from build123d import *

# Parameters (mm, degrees)
SKETCH1_R                = 200
BOSS_EXTRUDE1_DEPTH      = 15
BOSS_EXTRUDE2_DEPTH      = 200
CUT_EXTRUDE1_DEPTH       = 286.087705803
CUT_EXTRUDE1_DEPTH_BACK  = 286.087705803
SKETCH3_R                = 85
CUT_EXTRUDE2_DEPTH       = 451.079120005
CUT_EXTRUDE2_DEPTH_BACK  = 451.079120005
SKETCH4_R                = 11
CUT_EXTRUDE3_DEPTH       = 451.079120105
CUT_EXTRUDE3_DEPTH_BACK  = 110
CUT_EXTRUDE4_DEPTH       = 110
BOSS_EXTRUDE3_DEPTH      = 200
CUT_EXTRUDE5_DEPTH       = 286.087705815
CUT_EXTRUDE5_DEPTH_BACK  = 286.087705815
SKETCH7_OUTSIDE_W        = 515.59
SKETCH7_OUTSIDE_H        = 515.59
SKETCH7_OUTSIDE_R        = 200
SKETCH9_R                = 5.9
BOSS_EXTRUDE4_DEPTH      = 230
CUT_EXTRUDE6_DEPTH       = 190
CUT_EXTRUDE8_DEPTH       = 307.879455313
CUT_EXTRUDE8_DEPTH_BACK  = 307.879455313
SKETCH12_OUTSIDE_W       = 584.34
SKETCH12_OUTSIDE_H       = 524.34
SKETCH12_OUTSIDE_W_2     = 160.728506479
SKETCH12_OUTSIDE_H_2     = 57.445626466
BOSS_EXTRUDE5_DEPTH      = 190
CUT_EXTRUDE10_DEPTH      = 198.357534097
CUT_EXTRUDE10_DEPTH_BACK = 198.357534097
SKETCH20_W               = 10
SKETCH20_H               = 6
BOSS_EXTRUDE6_DEPTH      = 200
CUT_EXTRUDE9_DEPTH       = 237.718926518
CUT_EXTRUDE9_DEPTH_BACK  = 237.718926518
SKETCH15_R               = 85
CUT_EXTRUDE11_START      = 4.5
CUT_EXTRUDE11_DEPTH      = 6
CUT_EXTRUDE12_DEPTH      = 10
CUT_EXTRUDE13_DEPTH      = 10
SKETCH25_R               = 2.75
CUT_EXTRUDE14_DEPTH      = 100
SKETCH26_R               = 3.05
CUT_EXTRUDE15_DEPTH      = 12.1
FILLET1_R                = 5
CUT_EXTRUDE16_DEPTH      = 3
LPATTERN1_COUNT          = 3
LPATTERN1_PITCH          = 30
CUT_EXTRUDE17_DEPTH      = 3
LPATTERN2_COUNT          = 3
LPATTERN2_PITCH          = 30
BOSS_EXTRUDE7_START      = 12.1
BOSS_EXTRUDE7_DEPTH      = 12.1


# Read off the part's stored shape, not the designer's step: Cut-Extrude11
with BuildPart() as part:
    # Sketch1 → Boss-Extrude1 (new body)
    with BuildSketch(Plane(origin=(0, 0, 0), x_dir=(1, 0, 0), z_dir=(0, 1, 0))):
        with Locations(Location((0, 0, 0), (0, 0, 270))):
            Circle(SKETCH1_R)
    extrude(amount=BOSS_EXTRUDE1_DEPTH)

    # Sketch2 → Boss-Extrude2 (add, symmetric)
    with BuildSketch(Plane.XY):
        Polygon((-25, 50.707142143), (25, 50.707142143), (60, 15), (-60, 15), align=None)
    extrude(amount=BOSS_EXTRUDE2_DEPTH, both=True)

    # Sketch3 → Cut-Extrude1 (cut, two sides: drawn at the far end of the back side and taken through both)
    with BuildSketch(Plane(origin=(0, 15, 0), x_dir=(1, 0, 0), z_dir=(0, 1, 0)).offset(-CUT_EXTRUDE1_DEPTH_BACK)):
        with Locations(Location((0, 0, 0), (0, 0, 270))):
            Circle(SKETCH3_R)
    extrude(amount=CUT_EXTRUDE1_DEPTH + CUT_EXTRUDE1_DEPTH_BACK, mode=Mode.SUBTRACT)

    # Sketch4 → Cut-Extrude2 (cut, two sides: drawn at the far end of the back side and taken through both)
    with BuildSketch(Plane(origin=(0, 0, -200), x_dir=(-1, 0, 0), z_dir=(0, 0, -1)).offset(-CUT_EXTRUDE2_DEPTH_BACK)):
        with Locations((0, 29)):
            Circle(SKETCH4_R)
    extrude(amount=CUT_EXTRUDE2_DEPTH + CUT_EXTRUDE2_DEPTH_BACK, mode=Mode.SUBTRACT)

    # Sketch5 → Cut-Extrude3 (cut, two sides: drawn at the far end of the back side and taken through both)
    with BuildSketch(Plane.XY.offset(200).offset(-CUT_EXTRUDE3_DEPTH_BACK)):
        Polygon((-25, 50.707142143), (25, 50.707142143), (50.198039412, 25), (25, 25), (25, 15), (-25, 15), (-25, 25), (-50.198039412, 25), align=None)
    extrude(amount=CUT_EXTRUDE3_DEPTH + CUT_EXTRUDE3_DEPTH_BACK, mode=Mode.SUBTRACT)

    # Sketch6 → Cut-Extrude4 (cut)
    with BuildSketch(Plane(origin=(0, 0, -200), x_dir=(-1, 0, 0), z_dir=(0, 0, -1))):
        Polygon((-25, 50.707142143), (25, 50.707142143), (50.198039412, 25), (25, 25), (25, 15), (-25, 15), (-25, 25), (-50.198039412, 25), align=None)
    extrude(amount=-CUT_EXTRUDE4_DEPTH, mode=Mode.SUBTRACT)

    # Sketch8 → Boss-Extrude3 (add, symmetric)
    with BuildSketch(Plane(origin=(0, 0, 0), x_dir=(0, 0, -1), z_dir=(1, 0, 0))):
        Polygon((0, 15), (-30, 15), (-29.95, 44.999958333), (29.95, 44.999958333), (30, 15), align=None)
    extrude(amount=BOSS_EXTRUDE3_DEPTH, both=True)

    # Sketch7 outside → Cut-Extrude5 (cut, two sides: drawn at the far end of the back side and taken through both)
    with BuildSketch(Plane(origin=(0, 15, 0), x_dir=(1, 0, 0), z_dir=(0, 1, 0)).offset(-CUT_EXTRUDE5_DEPTH_BACK)):
        Rectangle(SKETCH7_OUTSIDE_W, SKETCH7_OUTSIDE_H)
        with Locations(Location((0, 0, 0), (0, 0, 97.180755781))):
            Circle(SKETCH7_OUTSIDE_R, mode=Mode.SUBTRACT)
    extrude(amount=CUT_EXTRUDE5_DEPTH + CUT_EXTRUDE5_DEPTH_BACK, mode=Mode.SUBTRACT)

    # Sketch9 → Boss-Extrude4 (add, symmetric)
    with BuildSketch(Plane(origin=(0, 0, 0), x_dir=(0, 0, -1), z_dir=(1, 0, 0))):
        with Locations(Location((0, 29, 0), (0, 0, 180))):
            Circle(SKETCH9_R)
    extrude(amount=BOSS_EXTRUDE4_DEPTH, both=True)

    # Sketch10 → Cut-Extrude6 (cut, symmetric)
    with BuildSketch(Plane(origin=(0, 0, 0), x_dir=(0, 0, -1), z_dir=(1, 0, 0))):
        Polygon((-30, 15), (30, 15), (29.95, 44.999958333), (-29.95, 44.999958333), align=None)
    extrude(amount=CUT_EXTRUDE6_DEPTH, both=True, mode=Mode.SUBTRACT)

    # Sketch12 outside → Cut-Extrude8 (cut, two sides: drawn at the far end of the back side and taken through both)
    with BuildSketch(Plane(origin=(0, 15, 0), x_dir=(1, 0, 0), z_dir=(0, 1, 0)).offset(-CUT_EXTRUDE8_DEPTH_BACK)):
        Rectangle(SKETCH12_OUTSIDE_W, SKETCH12_OUTSIDE_H)
        with Locations((-160.364253239, 0)):
            Rectangle(SKETCH12_OUTSIDE_W_2, SKETCH12_OUTSIDE_H_2, mode=Mode.SUBTRACT)
    extrude(amount=CUT_EXTRUDE8_DEPTH + CUT_EXTRUDE8_DEPTH_BACK, mode=Mode.SUBTRACT)

    # Sketch14 → Boss-Extrude5 (add)
    with BuildSketch(Plane(origin=(0, 0, 0), x_dir=(0, 0, -1), z_dir=(1, 0, 0))):
        Polygon((-28.722813233, 15), (-28.722813233, 35), (-18.722813233, 35), (-18.722813233, 25), (-10.722813233, 15), align=None)
        Polygon((28.722813233, 15), (28.722813233, 35), (18.722813233, 35), (18.722813233, 25), (10.722813233, 15), align=None)
    extrude(amount=-BOSS_EXTRUDE5_DEPTH)

    # Sketch16 → Cut-Extrude10 (cut, two sides: drawn at the far end of the back side and taken through both)
    with BuildSketch(Plane(origin=(-190, 0, 0), x_dir=(0, 0, -1), z_dir=(1, 0, 0)).offset(-CUT_EXTRUDE10_DEPTH_BACK)):
        Polygon((-28.722813233, 35), (-10.596657492, 40.452365235), (10.596657492, 40.452365235), (28.722813233, 35), (31.38249, 46.365203084), (-30.991256821, 46.365203084), align=None)
    extrude(amount=CUT_EXTRUDE10_DEPTH + CUT_EXTRUDE10_DEPTH_BACK, mode=Mode.SUBTRACT)

    # Sketch20 → Boss-Extrude6 (add)
    with BuildSketch(Plane(origin=(0, 0, 0), x_dir=(0, 0, -1), z_dir=(1, 0, 0))):
        with Locations((-33.722813233, 7.5)):
            Rectangle(SKETCH20_W, SKETCH20_H)
        with Locations((33.722813233, 7.5)):
            Rectangle(SKETCH20_W, SKETCH20_H)
    extrude(amount=-BOSS_EXTRUDE6_DEPTH)

    # Sketch15 → Cut-Extrude9 (cut, two sides: drawn at the far end of the back side and taken through both)
    with BuildSketch(Plane(origin=(0, 0, 0), x_dir=(1, 0, 0), z_dir=(0, 1, 0)).offset(-CUT_EXTRUDE9_DEPTH_BACK)):
        Circle(SKETCH15_R)
    extrude(amount=CUT_EXTRUDE9_DEPTH + CUT_EXTRUDE9_DEPTH_BACK, mode=Mode.SUBTRACT)

    # Cut-Extrude11 outline → Cut-Extrude11 (cut)
    with BuildSketch(Plane(origin=(0, 0, 0), x_dir=(1, 0, 0), z_dir=(0, 1, 0)).offset(CUT_EXTRUDE11_START)):
        with BuildLine():
            ThreePointArc((-196.215554265, -38.722813233), (-197.13457286, -33.733665434), (-197.926754129, -28.722813233))
            Line((-197.926754129, -28.722813233), (-200, -28.722813233))
            Line((-200, -28.722813233), (-200, -38.722813233))
            Line((-200, -38.722813233), (-196.215554265, -38.722813233))
        make_face()
        with BuildLine():
            Line((-200, 28.722813233), (-197.926754129, 28.722813233))
            ThreePointArc((-197.926754129, 28.722813233), (-197.13457286, 33.733665434), (-196.215554265, 38.722813233))
            Line((-196.215554265, 38.722813233), (-200, 38.722813233))
            Line((-200, 38.722813233), (-200, 28.722813233))
        make_face()
    extrude(amount=CUT_EXTRUDE11_DEPTH, mode=Mode.SUBTRACT)

    # Sketch23 → Cut-Extrude12 (cut)
    with BuildSketch(Plane(origin=(0, 0, -38.722813233), x_dir=(-1, 0, 0), z_dir=(0, 0, -1))):
        Polygon((75.667322771, 10.5), (80, 10.5), (90, 10.5), (90, 4.5), (75.667322771, 4.5), align=None)
    extrude(amount=-CUT_EXTRUDE12_DEPTH, mode=Mode.SUBTRACT)

    # Sketch24 → Cut-Extrude13 (cut)
    with BuildSketch(Plane.XY.offset(38.722813233)):
        Polygon((-75.667322771, 10.5), (-80, 10.5), (-90, 10.5), (-90, 4.5), (-75.667322771, 4.5), align=None)
    extrude(amount=-CUT_EXTRUDE13_DEPTH, mode=Mode.SUBTRACT)

    # Sketch25 → Cut-Extrude14 (cut)
    with BuildSketch(Plane.XY.offset(28.722813233)):
        with Locations((-167.926754129, 30)):
            Circle(SKETCH25_R)
        with Locations((-107.926754129, 30)):
            Circle(SKETCH25_R)
        with Locations((-137.926754129, 30)):
            Circle(SKETCH25_R)
    extrude(amount=-CUT_EXTRUDE14_DEPTH, mode=Mode.SUBTRACT)

    # Sketch26 → Cut-Extrude15 (cut)
    with BuildSketch(Plane.ZY.offset(230)):
        with Locations((0, 29)):
            Circle(SKETCH26_R)
    extrude(amount=-CUT_EXTRUDE15_DEPTH, mode=Mode.SUBTRACT)

    # Fillet1
    fillet1_edges = [part.edges().sort_by_distance(p)[0] for p in [
        (-199.912956058, 29, -5.9),
    ]]
    fillet(fillet1_edges, radius=FILLET1_R)

    # Sketch27 → Cut-Extrude16 (cut)
    with BuildSketch(Plane.XY.offset(-18.722813233)):
        Polygon((-167.926754129, 34.1), (-165.556754129, 34.1), (-163.060757334, 30), (-165.556754129, 25.9), (-167.926754129, 25.9), (-170.296754129, 25.9), (-172.663890233, 30), (-170.296754129, 34.1), align=None)
    cut_extrude16 = extrude(amount=-CUT_EXTRUDE16_DEPTH, mode=Mode.SUBTRACT)

    # LPattern1: Cut-Extrude16 ×3
    with Locations(*[(i * LPATTERN1_PITCH, 0, 0) for i in range(1, LPATTERN1_COUNT)]):
        add(cut_extrude16, mode=Mode.SUBTRACT)

    # Sketch28 → Cut-Extrude17 (cut)
    with BuildSketch(Plane(origin=(0, 0, 18.722813233), x_dir=(-1, 0, 0), z_dir=(0, 0, -1))):
        Polygon((107.926754129, 34.1), (110.296754129, 34.1), (112.663890233, 30), (110.296754129, 25.9), (107.926754129, 25.9), (105.556754129, 25.9), (103.189618025, 30), (105.556754129, 34.1), align=None)
    cut_extrude17 = extrude(amount=-CUT_EXTRUDE17_DEPTH, mode=Mode.SUBTRACT)

    # LPattern2: Cut-Extrude17 ×3
    with Locations(*[(-i * LPATTERN2_PITCH, 0, 0) for i in range(1, LPATTERN2_COUNT)]):
        add(cut_extrude17, mode=Mode.SUBTRACT)

    # Sketch29 → Boss-Extrude7 (add)
    with BuildSketch(Plane.ZY.offset(217.9).offset(BOSS_EXTRUDE7_START)):
        with BuildLine():
            Line((-1.673320053, 31.55), (1.673320053, 31.55))
            ThreePointArc((1.673320053, 31.55), (0, 32.05), (-1.673320053, 31.55))
        make_face()
    extrude(amount=-BOSS_EXTRUDE7_DEPTH)


solid = part.part
Geometry check sheet. Reference: the model listing, model coordinates, mm. A direction names the side the tool comes from. Give positions to 0.01 mm unless a question says otherwise; leave off trailing zeros. Loops run counter-clockwise (first coordinate to the right, second up) from the corner with the lowest first, then second, coordinate; pieces in that order, holes last.
(1) Section check C-C on z = 33.5. Record the cut outline in (x, y), then the cut area to 3 significant figures.
From the geometry:
outline: (-197.17, 4.5) - (-90, 4.5) - (-90, 10.5) - (-197.17, 10.5) - close
area: 643 mm2
(2) Section check A-A on x = -127.5. Record the cut outline in (y, z), then the cut area to 3 significant figures.
From the geometry:
outline: (0, -28.72) - (4.5, -28.72) - (4.5, -38.72) - (10.5, -38.72) - (10.5, -28.72) - (35, -28.72) - (35, -18.72) - (25, -18.72) - (15, -10.72) - (15, 10.72) - (25, 18.72) - (35, 18.72) - (35, 28.72) - (10.5, 28.72) - (10.5, 38.72) - (4.5, 38.72) - (4.5, 28.72) - (0, 28.72) - close
area: 1,460 mm2
(3) Section check B-B on z = -14.5. Record the cut outline in (x, y).
From the geometry:
outline: (-199.47, 0) - (-83.75, 0) - (-83.75, 19.72) - (-190, 19.72) - (-190, 39.28) - (-199.47, 39.28) - close
(4) Depth check by flat-ended pin: pin 1 Ø8 at (x, z) = (-210.5, -11.5) entering from +Y; pin 2 Ø1.5 at (x, y) = (-106, 13) entering from -Z; pin 3 Ø3 at (x, z) = (-155, -14.5) entering from +Y; pin 4 Ø1.5 at (x, z) = (-138, -19.5) entering from +Y. Enter the tip coordinate at first touch or a pass-through.
From the geometry:
pin 1: passes through
pin 2: stops at z = -28.72
pin 3: stops at y = 21.6
pin 4: stops at y = 35
(5) Release check for a two-part mould opening along X. For faces 1 (the cylindrical face through (-217.178, 24.025, 3.172)), 2 (the flat face through (-217.9, 29, 0)), 3 (the flat face through (-104.357, 32.021, 20.202)) record: released by +X, released by -X, zero draft, split by the parting line, or undercut.
From the geometry:
face 1: zero draft
face 2: released by -X
face 3: undercut
(6) Set-up check for faces 4 (the flat face through (-134, 35, -24)), 5 (the flat face through (-111.464, 27.921, -20.202)), 6 (the flat face through (-135.7, 34.5, 18.723)), 7 (the flat face through (-224, 31.55, 0)): record each of +Z, -Z, +X, -X, +Y, -Y from which the full face is reachable in a straight line by a thin tool's end or side.
From the geometry:
face 4: +Z, -Z, +X, +Y
face 5: none
face 6: +X, +Y
face 7: -X
(7) Thickness scan on L1, parallel to Z at x = -149.5, y = 27; L2, parallel to Y at x = -220.75, z = 0; L3, parallel to Z at x = -225, y = 29. Record the ranges inside material, lowest first.
From the geometry:
L1: z = -28.72 to -18.72, 18.72 to 28.72
L2: y = 23.1 to 25.95, 31.55 to 34.9
L3: z = -5.9 to -3.05, 3.05 to 5.9
